Verification items for the finished model (mm, model axes). A direction names the side the tool comes from. Coordinates: 2 decimals unless noted, no trailing zeros. Write each loop counter-clockwise with the first axis right and the second up, starting at its lowest first coordinate (ties: lowest second). Pieces come first, ordered by that corner, then holes.
```python
from build123d import *

# Parameters (mm, degrees)
SKETCH1_W           = 2.5
SKETCH1_H           = 8.5
BOSS_EXTRUDE1_DEPTH = 0.8
SKETCH2_W           = 2.5
SKETCH2_H           = 2.5
BOSS_EXTRUDE2_DEPTH = 0.6
SKETCH3_R           = 0.375
CUT_EXTRUDE1_DEPTH  = 0.2


with BuildPart() as part:
    # Sketch1 → Boss-Extrude1 (new body)
    with BuildSketch(Plane(origin=(0, 0, 0), x_dir=(1, 0, 0), z_dir=(0, 1, 0))):
        with Locations((1.25, 4.25)):
            Rectangle(SKETCH1_W, SKETCH1_H)
    extrude(amount=BOSS_EXTRUDE1_DEPTH)

    # Sketch2 → Boss-Extrude2 (add)
    with BuildSketch(Plane(origin=(0, 0.8, 0), x_dir=(1, 0, 0), z_dir=(0, 1, 0))):
        with Locations((1.25, 4.25)):
            Rectangle(SKETCH2_W, SKETCH2_H)
    extrude(amount=BOSS_EXTRUDE2_DEPTH)

    # Sketch3 → Cut-Extrude1 (cut)
    with BuildSketch(Plane(origin=(0, 1.4, 0), x_dir=(1, 0, 0), z_dir=(0, 1, 0))):
        with Locations((1.25, 4.25)):
            Circle(SKETCH3_R)
    extrude(amount=-CUT_EXTRUDE1_DEPTH, mode=Mode.SUBTRACT)


solid = part.part
```
1. Tool access check on faces 1 (the flat face through (1, 0.8, -2)), 2 (the flat face through (1, 0.8, -7)), 3 (the flat face through (1, 0, -4)). Record the directions out of +Z, -Z, +X, -X, +Y, -Y that give a thin tool (end or side, any length) a straight path to the whole face; none if there is none.
2. Sectioned sample at D-D, the plane x = 1.25. Record the boundary of the cut face in (y, z) (3 decimals), and give its area (3 significant figures).
3. Sectioned sample at B-B, the plane z = -4.25. Record the boundary of the cut face in (x, y) (3 decimals).
4. Sectioned sample at A-A, the plane x = 2.1. Record the boundary of the cut face in (y, z).
5. Sectioned sample at C-C, the plane y = 0.9. Record the boundary of the cut face in (x, z).
6. Material ranges on L1, parallel to X at y = 1.35, z = -4.25 (3 decimals); L2, parallel to Z at x = 1.25, y = 1.35 (3 decimals); L3, parallel to Z at x = 0.9, y = 1.1, recorded low to high.
Outcome:
1. face 1: +Z, +X, -X, +Y
1. face 2: -Z, +X, -X, +Y
1. face 3: +Z, -Z, +X, -X, -Y
2. outline: (0, -8.5) - (0.8, -8.5) - (0.8, -5.5) - (1.4, -5.5) - (1.4, -4.625) - (1.2, -4.625) - (1.2, -3.875) - (1.4, -3.875) - (1.4, -3) - (0.8, -3) - (0.8, 0) - (0, 0) - close
2. area: 8.15 mm2
3. outline: (0, 0) - (2.5, 0) - (2.5, 1.4) - (1.625, 1.4) - (1.625, 1.2) - (0.875, 1.2) - (0.875, 1.4) - (0, 1.4) - close
4. outline: (0, -8.5) - (0.8, -8.5) - (0.8, -5.5) - (1.4, -5.5) - (1.4, -3) - (0.8, -3) - (0.8, 0) - (0, 0) - close
5. outline: (0, -5.5) - (2.5, -5.5) - (2.5, -3) - (0, -3) - close
6. L1: x = 0 to 0.875, 1.625 to 2.5
6. L2: z = -5.5 to -4.625, -3.875 to -3
6. L3: z = -5.5 to -3
